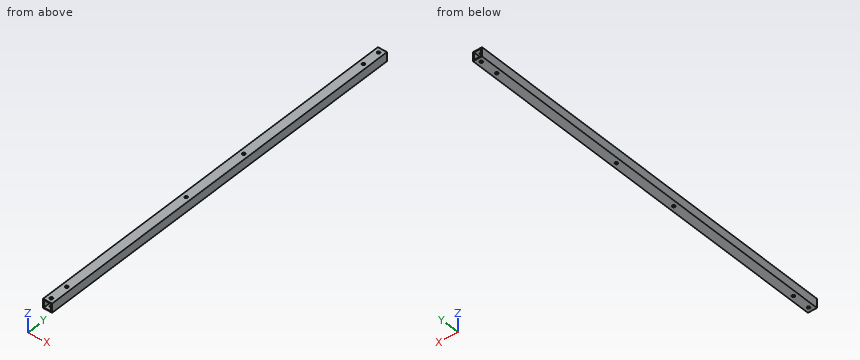
from build123d import *

# Parameters (mm, degrees)
SKETCH_1_W          = 10
SKETCH_1_H          = 10
SKETCH_1_W_2        = 8
SKETCH_1_H_2        = 8
EXTRUDE_1_DEPTH     = 218.715
SKETCH_2_R          = 1.6
CUT_EXTRUDE_1_DEPTH = 213.715
SKETCH_3_R          = 1.6
CUT_EXTRUDE_2_DEPTH = 10


with BuildPart() as part:
    # ｽｹｯﾁ1 → ﾎﾞｽ - 押し出し1 (new, symmetric)
    with BuildSketch(Plane(origin=(0, 0, 0), x_dir=(1, 0, 0), z_dir=(0, 1, 0))):
        Rectangle(SKETCH_1_W, SKETCH_1_H)
        Rectangle(SKETCH_1_W_2, SKETCH_1_H_2, mode=Mode.SUBTRACT)
    extrude(amount=EXTRUDE_1_DEPTH, both=True)

    # ｽｹｯﾁ2 → ｶｯﾄ - 押し出し1 (cut, symmetric)
    with BuildSketch(Plane.XY.offset(5)):
        with Locations((0, 213.715)):
            Circle(SKETCH_2_R)
        with Locations((0, 193.715)):
            Circle(SKETCH_2_R)
    cut_extrude_1 = extrude(amount=CUT_EXTRUDE_1_DEPTH, both=True, mode=Mode.SUBTRACT)

    # ﾐﾗｰ1: ｶｯﾄ - 押し出し1 across plane
    add(cut_extrude_1.mirror(Plane.ZX), mode=Mode.SUBTRACT)

    # ｽｹｯﾁ3 → ｶｯﾄ - 押し出し2 (cut)
    with BuildSketch(Plane.XY.offset(5)):
        with Locations((0.004997943, -37.579217745)):
            Circle(SKETCH_3_R)
        with Locations((-1.455e-06, 37.420782255)):
            Circle(SKETCH_3_R)
    extrude(amount=-CUT_EXTRUDE_2_DEPTH, mode=Mode.SUBTRACT)


solid = part.part
The model under review builds one solid part; all positions refer to its coordinate system, in mm. Round coordinates to 2 decimals unless told otherwise and drop trailing zeros. Write each loop counter-clockwise with the first axis right and the second up, starting at its lowest first coordinate (ties: lowest second). Pieces come first, ordered by that corner, then holes. Notation, with made-up numbers: (22, -13.75) - (31, -13.75) arc R14 cw to (31, 2.25) - close; hole circle Ø4 at (21, -27.75). An arc over 180 degrees is marked (long way). One line per item, written item: value. Start each with the question number.
1. Consider section B-B on y = 105.5. Write out the cut boundary in (x, z), and give its area (3 significant figures).
2. To check wall thickness, follow L1, parallel to X at y = -128.5, z = 1.25. State the ranges of the line that lie inside material, in increasing order. Write a range as from..to.
3. Clearance check with flat-ended pins moving along their axes: P1, Ø4, axis at x = 3, z = -2, coming from the -Y side (3 decimals); P2, Ø1, axis at x = 2, z = -1.5, coming from the +Y side (1 decimal). State where each tip first meets the part, or that it passes through.
4. Consider section A-A on z = 2. Write out the cut boundary in (x, y) (3 decimals).
5. Consider section C-C on x = 0. State how many separate pieces and enclosed holes the cut face has, and give its area (3 significant figures).
Checks:
1. outline: (-5, -5) - (5, -5) - (5, 5) - (-5, 5) - close; hole (-4, -4) - (4, -4) - (4, 4) - (-4, 4) - close
1. area: 36.0 mm^2
2. L1: x = -5..-4, 4..5
3. P1: stops at y = -218.715
3. P2: passes through
4. outline: (-5, -218.715) - (-4, -218.715) - (-4, 218.715) - (-5, 218.715) - close; (4, -218.715) - (5, -218.715) - (5, 218.715) - (4, 218.715) - close
5. separate pieces: 14
5. enclosed holes: 0
5. area: 836 mm^2
